Geometry check sheet. Reference: drawing and pictorial views, mm from the part's lowest x, y, z. Give positions to 0.01 mm unless a question says otherwise; leave off trailing zeros. Loops run counter-clockwise (first coordinate to the right, second up) from the corner with the lowest first, then second, coordinate; pieces in that order, holes last. Notation, with made-up numbers: M 46.5,81.5 L 87.5,81.5 A20 cw 87.5,106.5 Z; hole C -32,68 d11. An arc over 180 degrees is marked long. Put each result on its own line as item: value. Start each with the question number.
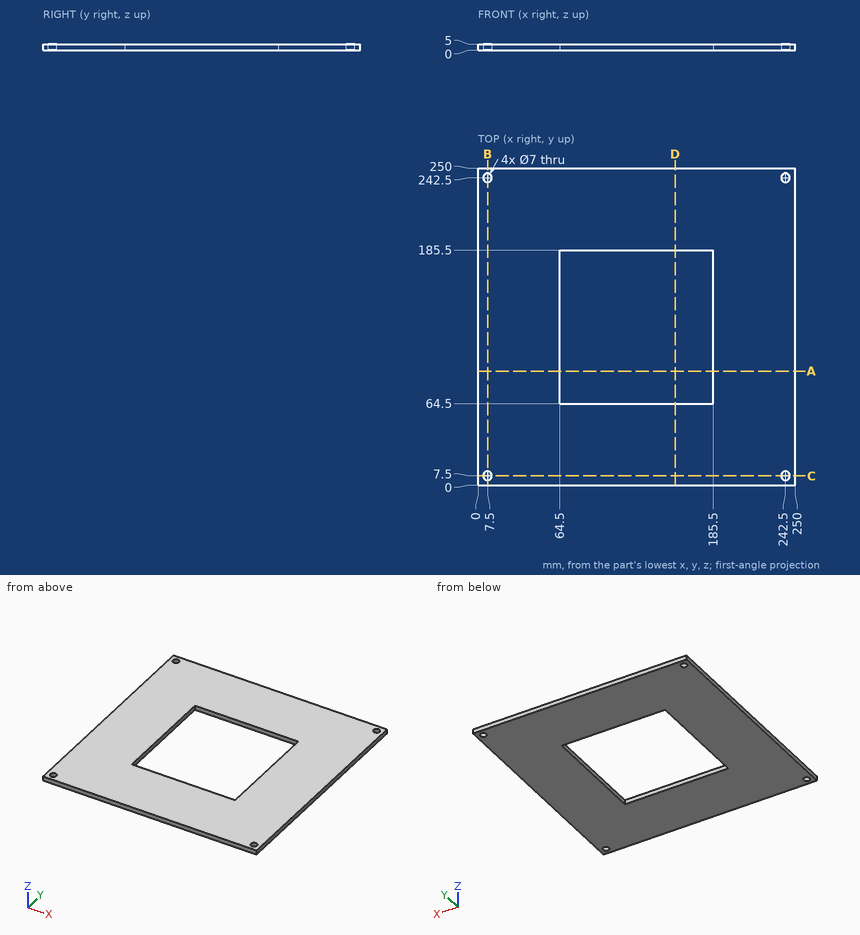
Q1. Depth check by flat-ended pin: P1, Ø6.5, axis at x = 7.5, y = 242.5, coming from the +Z side. Enter the tip coordinate at first touch or a pass-through.
Q2. Section check B-B, the plane x = 7.5. Record the cut outline in (y, z).
Q3. Section check A-A, the plane y = 90. Record the cut outline in (x, z), then the cut area to 3 significant figures.
Q4. Thickness scan on line 1 along Y through (x, z) = (7.5, 3.6); line 2 along X through (y, z) = (178.5, 4.65). Record the ranges inside material, lowest first. Write a range as [from, to].
Found:
1. P1: passes through
2. outline: M 0,0 L 4,0 L 4,5 L 0,5 Z; M 11,0 L 239,0 L 239,5 L 11,5 Z; M 246,0 L 250,0 L 250,5 L 246,5 Z
3. outline: M 0,0 L 64.5,0 L 64.5,5 L 0,5 Z; M 185.5,0 L 250,0 L 250,5 L 185.5,5 Z
3. area: 645 mm^2
4. line 1: y = [0, 4], [11, 239], [246, 250]
4. line 2: x = [0, 64.5], [185.5, 250]
